Geometry check sheet. Reference: the model listing, model coordinates, mm. Give positions to 0.01 mm unless a question says otherwise; leave off trailing zeros. Write each loop counter-clockwise with the first axis right and the second up, starting at its lowest first coordinate (ties: lowest second). Pieces come first, ordered by that corner, then holes. Notation, with made-up numbers: (73.25, 37) - (129.25, 37) arc R13 ccw to (129.25, 58) - close; hole circle Ø4 at (-28.5, 0). An arc over 180 degrees is marked (long way). Use a Markdown table: item, result.
```python
from build123d import *

# Parameters (mm, degrees)
SKETCH1_W           = 50
SKETCH1_H           = 70
BOSS_EXTRUDE1_DEPTH = 5
SKETCH2_R           = 1.6
CUT_EXTRUDE1_DEPTH  = 10


with BuildPart() as part:
    # Sketch1 → Boss-Extrude1 (new body)
    with BuildSketch(Plane(origin=(0, 0, 0), x_dir=(1, 0, 0), z_dir=(0, 1, 0))):
        with Locations((-4.575074469, 3.274395374)):
            Rectangle(SKETCH1_W, SKETCH1_H)
        with BuildLine():
            Line((-25.838530436, 31.787851342), (16.688381499, 31.787851342))
            ThreePointArc((16.688381499, 31.787851342), (18.938381499, 29.537851342), (16.688381499, 27.287851342))
            Line((16.688381499, 27.287851342), (-25.838530436, 27.287851342))
            ThreePointArc((-25.838530436, 27.287851342), (-28.088530436, 29.537851342), (-25.838530436, 31.787851342))
        make_face(mode=Mode.SUBTRACT)
        with BuildLine():
            Line((-9.575074469, 18.274395374), (0.424925531, 18.274395374))
            ThreePointArc((0.424925531, 18.274395374), (5.424925531, 13.274395374), (0.424925531, 8.274395374))
            Line((0.424925531, 8.274395374), (-9.575074469, 8.274395374))
            ThreePointArc((-9.575074469, 8.274395374), (-14.575074469, 13.274395374), (-9.575074469, 18.274395374))
        make_face(mode=Mode.SUBTRACT)
        with BuildLine():
            Line((-25.838530436, -5.239060593), (16.688381499, -5.239060593))
            ThreePointArc((16.688381499, -5.239060593), (18.938381499, -2.989060593), (16.688381499, -0.739060593))
            Line((16.688381499, -0.739060593), (-25.838530436, -0.739060593))
            ThreePointArc((-25.838530436, -0.739060593), (-28.088530436, -2.989060593), (-25.838530436, -5.239060593))
        make_face(mode=Mode.SUBTRACT)
    extrude(amount=BOSS_EXTRUDE1_DEPTH)

    # Sketch2 → Cut-Extrude1 (cut)
    with BuildSketch(Plane.XY.offset(31.725604626)):
        with Locations((-4.575074469, 2.5)):
            Circle(SKETCH2_R)
        with Locations((-19.575074469, 2.5)):
            Circle(SKETCH2_R)
        with Locations((10.424925531, 2.5)):
            Circle(SKETCH2_R)
    extrude(amount=-CUT_EXTRUDE1_DEPTH, mode=Mode.SUBTRACT)


solid = part.part
```
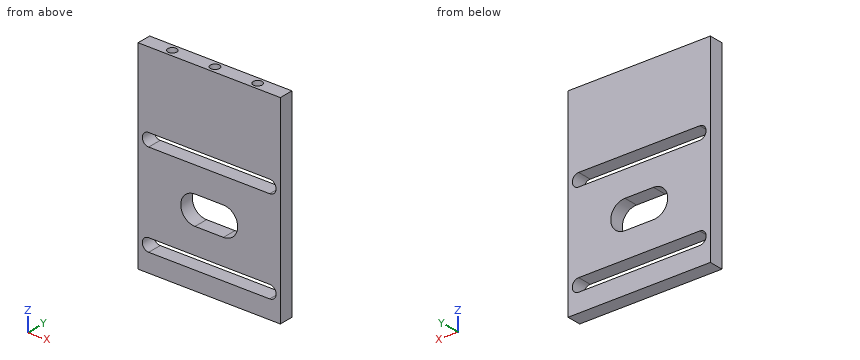
1) Section check D-D on x = -5. Record the boundary of the cut face in (y, z), then the cut area to 3 significant figures.
Working result:
| item | result |
|---|---|
| outline | (0, -38.27) - (5, -38.27) - (5, -31.79) - (0, -31.79) - close; (0, -27.29) - (5, -27.29) - (5, -18.27) - (0, -18.27) - close; (0, -8.27) - (5, -8.27) - (5, 0.74) - (0, 0.74) - close; (0, 5.24) - (5, 5.24) - (5, 31.73) - (4.04, 31.73) - (4.04, 21.73) - (0.96, 21.73) - (0.96, 31.73) - (0, 31.73) - close |
| area | 224 mm² |
2) Depth check by flat-ended pin: P1, Ø1, axis at x = -19, y = 3, coming from the +Z side; P2, Ø12, axis at x = -9.5, z = 19.5, coming from the -Y side. Enter the tip coordinate at first touch or a pass-through.
Working result:
| item | result |
|---|---|
| P1 | stops at z = 21.73 |
| P2 | stops at y = 0 |
3) Section check A-A on z = 25. Record the boundary of the cut face in (x, y).
Working result:
| item | result |
|---|---|
| outline | (-29.58, 0) - (20.42, 0) - (20.42, 5) - (-29.58, 5) - close; hole circle Ø3.2 at (-19.58, 2.5); hole circle Ø3.2 at (-4.58, 2.5); hole circle Ø3.2 at (10.42, 2.5) |
4) Section check B-B on y = 2.5. Record the boundary of the cut face in (x, z).
Working result:
| item | result |
|---|---|
| outline | (-29.58, -38.27) - (20.42, -38.27) - (20.42, 31.73) - (12.02, 31.73) - (12.02, 21.73) - (8.82, 21.73) - (8.82, 31.73) - (-2.98, 31.73) - (-2.98, 21.73) - (-6.18, 21.73) - (-6.18, 31.73) - (-17.98, 31.73) - (-17.98, 21.73) - (-21.18, 21.73) - (-21.18, 31.73) - (-29.58, 31.73) - close; hole (-25.84, -31.79) - (16.69, -31.79) arc R2.25 ccw to (16.69, -27.29) - (-25.84, -27.29) arc R2.25 ccw to start; hole (-25.84, 0.74) - (16.69, 0.74) arc R2.25 ccw to (16.69, 5.24) - (-25.84, 5.24) arc R2.25 ccw to start; hole (-9.58, -18.27) - (0.42, -18.27) arc R5 ccw to (0.42, -8.27) - (-9.58, -8.27) arc R5 ccw to start |
5) Material ranges on L1, parallel to Z at x = 13, y = 3.4; L2, parallel to Z at x = -20, y = 1.5; L3, parallel to Z at x = 0.5, y = 0.7, recorded low to high. Write a range as from..to.
Working result:
| item | result |
|---|---|
| L1 | z = -38.27..-31.79, -27.29..0.74, 5.24..31.73 |
| L2 | z = -38.27..-31.79, -27.29..0.74, 5.24..21.73 |
| L3 | z = -38.27..-31.79, -27.29..-18.27, -8.27..0.74, 5.24..31.73 |
6) Section check C-C on x = -12.5. Record the boundary of the cut face in (y, z), then the cut area to 3 significant figures.
Working result:
| item | result |
|---|---|
| outline | (0, -38.27) - (5, -38.27) - (5, -31.79) - (0, -31.79) - close; (0, -27.29) - (5, -27.29) - (5, -17.33) - (0, -17.33) - close; (0, -9.22) - (5, -9.22) - (5, 0.74) - (0, 0.74) - close; (0, 5.24) - (5, 5.24) - (5, 31.73) - (0, 31.73) - close |
| area | 264 mm² |
